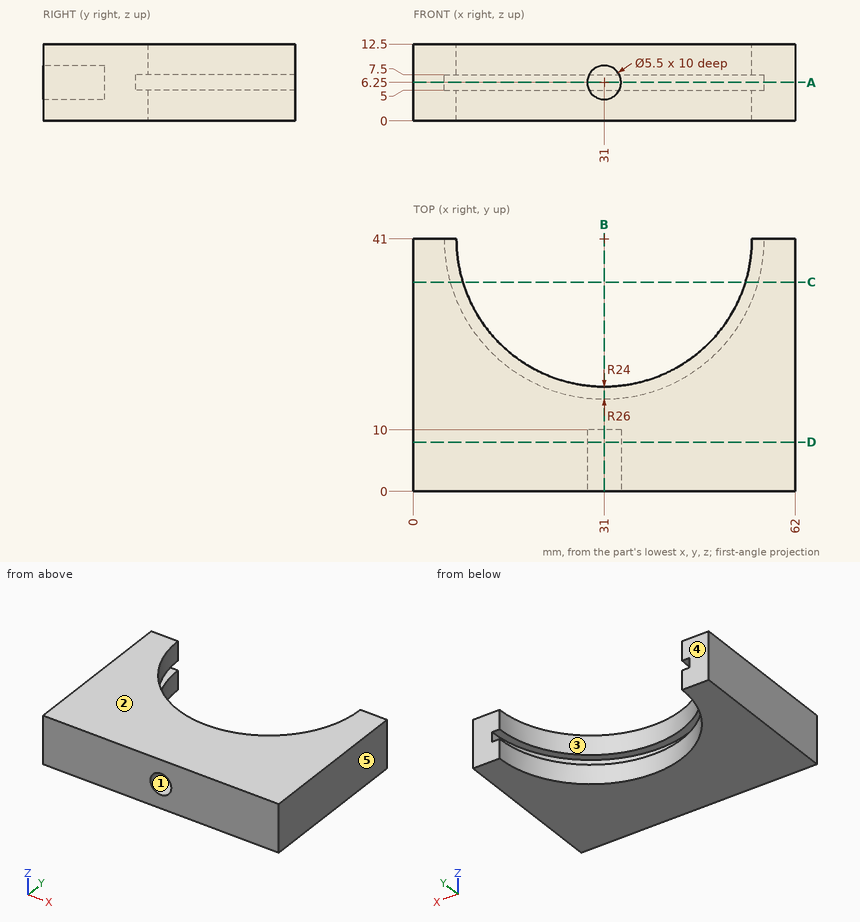
Print and shaded views of the part. All mm, measured from the part's lowest x, y and z. A direction names the side the tool comes from. Give positions to 0.01 mm unless a question says otherwise; leave off trailing zeros. Loops run counter-clockwise (first coordinate to the right, second up) from the corner with the lowest first, then second, coordinate; pieces in that order, holes last. Notation, with made-up numbers: (37, 69) - (43, 69) arc R15 cw to (43, 97) - close; hole circle Ø5 at (-31, 71). An arc over 180 degrees is marked (long way). Use a Markdown table: item, result.
(1) Which spindle directions (+Z, -Z, +X, -X, +Y, -Y) get a long thin tool onto all of the face, cutting with end or side? Do the marked faces 1 and 2. Say none if no direction does.
Taken from the geometry:
| item | result |
|---|---|
| face 1 | -Y |
| face 2 | +Z, +X, -X, +Y, -Y |
(2) Drop flat-ended pins along their axis: pin 1 Ø21 at (x, y) = (20.5, 30) entering from -Z; pin 2 Ø5 at (x, z) = (31, 6.25) entering from -Y; pin 3 Ø1 at (x, z) = (12, 2) entering from +Y. Give the stop position or say it passes through.
Taken from the geometry:
| item | result |
|---|---|
| pin 1 | z = 0 |
| pin 2 | y = 10 |
| pin 3 | y = 27.01 |
(3) Band-saw the part on C-C (y = 34). Give the cut face in (x, z), and give its area (3 significant figures).
Taken from the geometry:
| item | result |
|---|---|
| outline | (0, 0) - (8.04, 0) - (8.04, 5) - (5.96, 5) - (5.96, 7.5) - (8.04, 7.5) - (8.04, 12.5) - (0, 12.5) - close; (53.96, 0) - (62, 0) - (62, 12.5) - (53.96, 12.5) - (53.96, 7.5) - (56.04, 7.5) - (56.04, 5) - (53.96, 5) - close |
| area | 191 mm2 |
(4) Band-saw the part on B-B (x = 31). Give the cut face in (y, z).
Taken from the geometry:
| item | result |
|---|---|
| outline | (0, 0) - (17, 0) - (17, 5) - (15, 5) - (15, 7.5) - (17, 7.5) - (17, 12.5) - (0, 12.5) - (0, 9) - (10, 9) - (10, 3.5) - (0, 3.5) - close |
(5) Wall check: line 1 along X through (y, z) = (7.25, 6.25); line 2 along X through (y, z) = (4, 7.5); line 3 along Y through (x, z) = (14, 8.5). Give the ranges that are in metal, low to high.
Taken from the geometry:
| item | result |
|---|---|
| line 1 | 0 to 28.25, 33.75 to 62 |
| line 2 | 0 to 28.55, 33.45 to 62 |
| line 3 | 0 to 24.06 |
(6) Band-saw the part on A-A (z = 6.25). Give the cut face in (x, y), and give its area (3 significant figures).
Taken from the geometry:
| item | result |
|---|---|
| outline | (0, 0) - (28.25, 0) - (28.25, 10) - (33.75, 10) - (33.75, 0) - (62, 0) - (62, 41) - (57, 41) arc R26 cw to (5, 41) - (0, 41) - close |
| area | 1,430 mm2 |
(7) Band-saw the part on D-D (y = 8). Give the cut face in (x, z).
Taken from the geometry:
| item | result |
|---|---|
| outline | (0, 0) - (62, 0) - (62, 12.5) - (0, 12.5) - close; hole circle Ø5.5 at (31, 6.25) |
(8) Pull direction X, two halves, no side cores. Call the marked faces 3, 4 and 5: +X half, -X half, draft (parallel to the pull), parting line (faces both ways), or undercut.
Taken from the geometry:
| item | result |
|---|---|
| face 3 | undercut |
| face 4 | draft |
| face 5 | +X half |
